The figure shows three views and two pictorial views of one solid part (mm, origin at its lowest corner). Answer the questions. Round coordinates to 2 decimals unless told otherwise and drop trailing zeros. Order: outer loops, then holes, each group sorted by start corner. A loop starts at its lowest first (then second) coordinate and runs counter-clockwise, first axis right, second up. Notation, with made-up numbers: (-30, 70.25) - (10, 70.25) arc R15 ccw to (10, 84.25) - close; hole circle Ø4 at (39.5, -26). An arc over 180 degrees is marked (long way). Answer as a JSON object with one key per item and string values. Group by question number.
Q1. A cutting plane is placed at C-C on z = 175. Determine the outline of the cut face in (x, y) (1 decimal).
Q2. Consider line 1 (X direction, y = 5.5, z = 170) (1 decimal); line 2 (Y direction, x = 286.75, z = 152.4) (1 decimal); line 3 (Z direction, x = 152.4, y = 1.95). Determine where each line is inside the solid, lowest interval first.
Q3. A cutting plane is placed at B-B on y = 34. Count the separate pieces of the cut face and the enclosed holes in it, and give its area (3 significant figures).
Q4. The mould has two halves that part along X. Classify the marked faces 1, 2, 3 and 4: pulls with the +X half, pulls with the -X half, needs draft (parallel to the pull), parting line crosses it, or undercut.
Q5. Given pin 1 Ø12 at (x, y) = (165.5, 11) entering from -Z; pin 2 Ø19 at (y, z) = (15, 139.5) entering from -X (1 decimal); pin 3 Ø1 at (x, y) = (267, 1) entering from +Z; pin 4 Ø3.5 at (x, y) = (47, 2) entering from +Z (1 decimal), each flat-ended and moving along its own axis, determine where each tip first touches the part or whether it passes through.
Q6. A cutting plane is placed at A-A on x = 152.4. Determine the outline of the cut face in (y, z) (1 decimal).
Q7. A cutting plane is placed at D-D on z = 254. Determine the outline of the cut face in (x, y) (1 decimal).
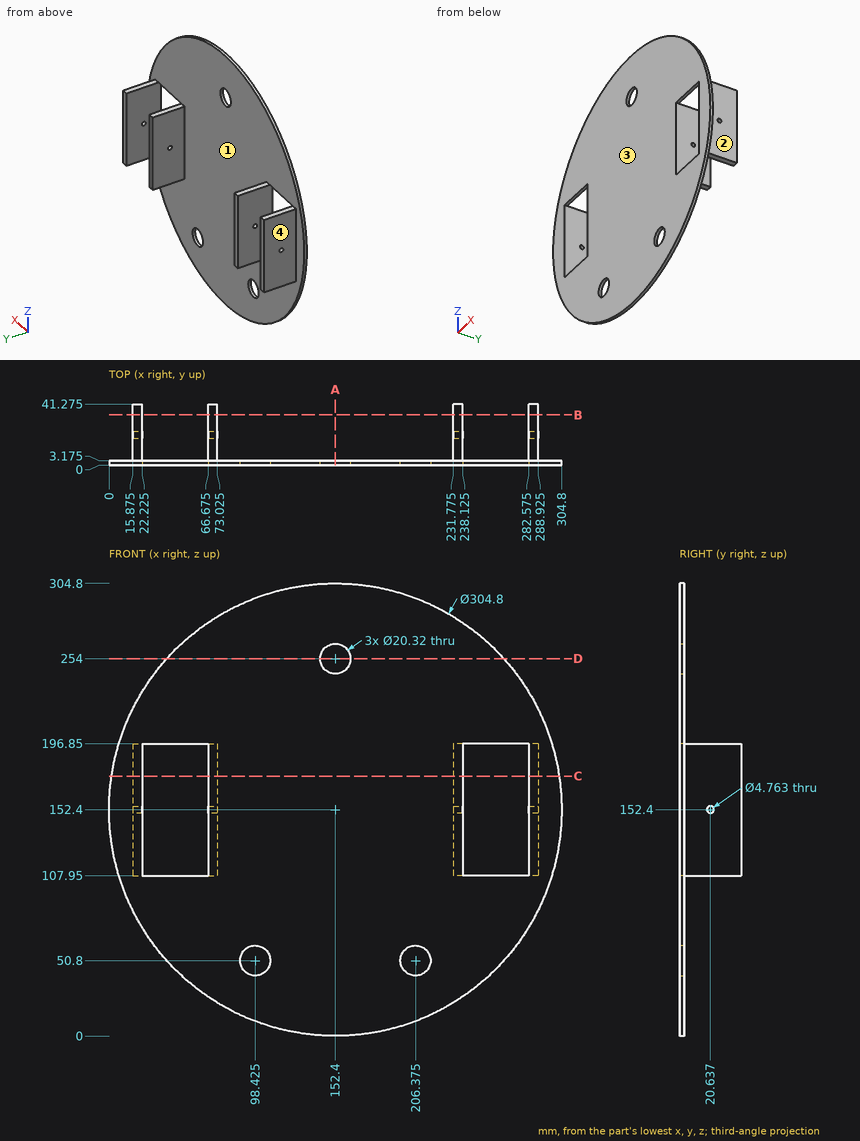
Result set:
{
 "1": {"outline": "(1.7, 0) - (22.2, 0) - (22.2, 41.3) - (15.9, 41.3) - (15.9, 3.2) - (1.7, 3.2) - close; (66.7, 0) - (238.1, 0) - (238.1, 41.3) - (231.8, 41.3) - (231.8, 3.2) - (73, 3.2) - (73, 41.3) - (66.7, 41.3) - close; (282.6, 0) - (303.1, 0) - (303.1, 3.2) - (288.9, 3.2) - (288.9, 41.3) - (282.6, 41.3) - close"},
 "2": {"line 1": "x = 15.9 to 22.2, 66.7 to 73, 231.8 to 238.1, 282.6 to 288.9", "line 2": "y = 0 to 18.3, 23 to 41.3", "line 3": "z = 0 to 243.84, 264.16 to 304.8"},
 "3": {"separate pieces": "4", "enclosed holes": "0", "area": "2,260 mm²"},
 "4": {"face 1": "undercut", "face 2": "pulls with the +X half", "face 3": "needs draft", "face 4": "pulls with the -X half"},
 "5": {"pin 1": "passes through", "pin 2": "stops at x = 15.9", "pin 3": "stops at z = 253.43", "pin 4": "stops at z = 264.1"},
 "6": {"outline": "(0, 0) - (3.2, 0) - (3.2, 243.8) - (0, 243.8) - close; (0, 264.2) - (3.2, 264.2) - (3.2, 304.8) - (0, 304.8) - close"},
 "7": {"outline": "(38.8, 0) - (142.2, 0) - (142.2, 3.2) - (38.8, 3.2) - close; (162.6, 0) - (266, 0) - (266, 3.2) - (162.6, 3.2) - close"}
}
